Source: CAD feature listing. Evaluate the final solid. Frame: model axes, mm. A direction names the side the tool comes from. Give positions to 0.01 mm unless a question says otherwise; leave off trailing zeros. Order: outer loops, then holes, each group sorted by start corner. A loop starts at its lowest first (then second) coordinate and runs counter-clockwise, first axis right, second up. Notation, with made-up numbers: M 84.5,48.5 L 122.5,48.5 A10 cw 122.5,67.5 Z; hole C 26,32 d5. An arc over 180 degrees is marked long. Answer as a JSON object with one key per item and string values. Group by question number.
1. Pull-direction query (X, two-part tool) for faces 1 (the cylindrical face through (-9.918, 17.785, -252.536)), 2 (the flat face through (-8, 3, -85.725)), 3 (the cylindrical face through (-25.78, 18.78, -183.78)), 4 (the flat face through (4.445, 19, -248)); classes: +X half, -X half, draft (parallel to the pull), parting line (faces both ways), or undercut.
2. Material intervals for L1, parallel to X at y = 10, z = -203.2; L2, parallel to Z at x = -7, y = 4 (3 decimals); L3, parallel to X at y = 32, z = -1, sorted ascending. Write a range as [from, to].
3. Section query B-B (z = -203.2). Output: boundary loops of the cut face in (x, y), plus the area to 3 significant figures.
4. Section query D-D (y = 33). Output: boundary loops of the cut face in (x, z) (3 decimals), plus the area to 3 significant figures.
5. Section query C-C (x = 0). Output: boundary loops of the cut face in (y, z) (3 decimals), plus the area to 3 significant figures.
6. Section query A-A (y = 19.05). Output: boundary loops of the cut face in (x, z) (3 decimals), plus the area to 3 significant figures.
7. Set-up query: faces 5 (the flat face through (-4.445, 19, -248)), 6 (the flat face through (-15.24, 19, -260)), 7 (the flat face through (-4.762, 3, -67)). Return all of +Z, -Z, +X, -X, +Y, -Y with unobstructed straight access to the full face (end or side cutting, diameter ignored); none if empty.
8. Pin query (flat end, axial travel): P1, Ø5.5, axis at y = 2, z = -73, coming from the -X side; P2, Ø1, axis at y = 5.5, z = -170, coming from the +X side; P3, Ø8, axis at y = 18, z = -218.5, coming from the +X side. Return the tip coordinate at first contact, or that it passes through.
from build123d import *

# Parameters (mm, degrees)
SKETCH2_R           = 12.827
BOSS_EXTRUDE1_DEPTH = 38.1
CUT_EXTRUDE1_REACH  = 283.22
SKETCH3_R           = 3.302
SKETCH4_W           = 23.114
SKETCH4_H           = 31.75
CUT_EXTRUDE2_DEPTH  = 5.08
SKETCH5_W           = 9.525
SKETCH5_H           = 38.1
CUT_EXTRUDE3_DEPTH  = 5.08
CUT_EXTRUDE4_REACH  = 281.078
SKETCH6_W           = 6.604
SKETCH6_H           = 3.429


with BuildPart() as part:
    # Sketch2 → Boss-Extrude1 (new body)
    with BuildSketch(Plane(origin=(0, 0, 0), x_dir=(1, 0, 0), z_dir=(0, 1, 0))):
        with BuildLine():
            Line((-25.4, 0), (-25.4, 181.02040352))
            ThreePointArc((-25.4, 181.02040352), (-25.79242718, 183.816851484), (-26.939393939, 186.397275394))
            ThreePointArc((-26.939393939, 186.397275394), (-31.231288537, 208.915690363), (-19.242424242, 228.45453641))
            ThreePointArc((-19.242424242, 228.45453641), (-16.295425059, 232.026851209), (-15.24, 236.535988061))
            Line((-15.24, 236.535988061), (-15.24, 274.635988061))
            Line((-15.24, 274.635988061), (-4.445, 274.635988061))
            Line((-4.445, 274.635988061), (-4.445, 221.33211339))
            ThreePointArc((-4.445, 221.33211339), (0, 184.531), (4.445, 221.33211339))
            Line((4.445, 221.33211339), (4.445, 274.635988061))
            Line((4.445, 274.635988061), (15.24, 274.635988061))
            Line((15.24, 274.635988061), (15.24, 236.535988061))
            ThreePointArc((15.24, 236.535988061), (16.295425059, 232.026851209), (19.242424242, 228.45453641))
            ThreePointArc((19.242424242, 228.45453641), (31.231288537, 208.915690363), (26.939393939, 186.397275394))
            ThreePointArc((26.939393939, 186.397275394), (25.79242718, 183.816851484), (25.4, 181.02040352))
            Line((25.4, 181.02040352), (25.4, 0))
            ThreePointArc((25.4, 0), (0, -25.4), (-25.4, 0))
        make_face()
        with Locations(Location((0, 0, 0), (0, 0, 90))):
            Circle(SKETCH2_R, mode=Mode.SUBTRACT)
    extrude(amount=BOSS_EXTRUDE1_DEPTH)

    # Cut-Extrude1: up to this face of the body (flat: up to its plane)
    cut_extrude1_end = Plane(part.part.faces().sort_by_distance((15.24, 19.05, -255.585988061))[0])
    # Sketch3 → Cut-Extrude1 (cut, up to the picked face)
    with BuildSketch(Plane.ZY.offset(15.24), mode=Mode.PRIVATE) as cut_extrude1_sk1:
        with Locations((-255.585988061, 19.05)):
            Circle(SKETCH3_R)
    cut_extrude1_tool1 = split(extrude(cut_extrude1_sk1.sketch, amount=-CUT_EXTRUDE1_REACH, mode=Mode.PRIVATE), bisect_by=cut_extrude1_end, keep=Keep.BOTH, mode=Mode.PRIVATE)
    add(cut_extrude1_tool1.solids().sort_by(Axis((-15.24, 19.05, -255.585988), (1, 0, 0)))[0], mode=Mode.SUBTRACT)

    # Sketch4 → Cut-Extrude2 (cut)
    with BuildSketch(Plane.XZ):
        with Locations((0, -101.6)):
            Rectangle(SKETCH4_W, SKETCH4_H)
    extrude(amount=-CUT_EXTRUDE2_DEPTH, mode=Mode.SUBTRACT)

    # Sketch5 → Cut-Extrude3 (cut)
    with BuildSketch(Plane.XZ):
        with Locations((0, -66.675)):
            Rectangle(SKETCH5_W, SKETCH5_H)
    extrude(amount=-CUT_EXTRUDE3_DEPTH, mode=Mode.SUBTRACT)

    # Sketch6 → Cut-Extrude4 (cut, up to next)
    with BuildSketch(Plane.XZ, mode=Mode.PRIVATE) as cut_extrude4_sk1:
        with Locations((0, -14.109205523)):
            Rectangle(SKETCH6_W, SKETCH6_H)
    cut_extrude4_tool1 = extrude(cut_extrude4_sk1.sketch, amount=-CUT_EXTRUDE4_REACH, mode=Mode.PRIVATE) & part.part
    add(cut_extrude4_tool1.solids().sort_by_distance((0, 0, -14.109206))[0], mode=Mode.SUBTRACT)


solid = part.part
Answer sheet:
{
 "1": {"face 1": "draft", "face 2": "undercut", "face 3": "-X half", "face 4": "undercut"},
 "2": {"L1": "[-31.75, -18.67], [18.67, 31.75]", "L2": "[-274.636, -220.507], [-185.893, -117.475], [-85.725, -10.749], [10.749, 24.416]", "L3": "[-25.4, -12.79], [12.79, 25.4]"},
 "3": {"outline": "M -31.75,0 L -18.67,0 L -18.67,38.1 L -31.75,38.1 Z; M 18.67,0 L 31.75,0 L 31.75,38.1 L 18.67,38.1 Z", "area": "997 mm^2"},
 "4": {"outline": "M -26.939,-186.397 A31.75 ccw -19.242,-228.455 A10.16 cw -15.24,-236.536 L -15.24,-274.636 L -4.445,-274.636 L -4.445,-221.332 A18.669 cw long 4.445,-221.332 L 4.445,-274.636 L 15.24,-274.636 L 15.24,-236.536 A10.16 cw 19.242,-228.455 A31.75 ccw 26.939,-186.397 A10.16 cw 25.4,-181.02 L 25.4,0 A25.4 ccw -25.4,0 L -25.4,-181.02 A10.16 cw Z; hole M -3.302,-15.824 L 3.302,-15.824 L 3.302,-12.395 A12.827 ccw long -3.302,-12.395 Z", "area": "12,200 mm^2"},
 "5": {"outline": "M 0,-184.531 L 38.1,-184.531 L 38.1,-15.824 L 0,-15.824 L 0,-47.625 L 5.08,-47.625 L 5.08,-117.475 L 0,-117.475 Z; M 0,12.827 L 38.1,12.827 L 38.1,25.4 L 0,25.4 Z", "area": "6,550 mm^2"},
 "6": {"outline": "M -26.939,-186.397 A31.75 ccw -19.242,-228.455 A10.16 cw -15.24,-236.536 L -15.24,-252.284 L -4.445,-252.284 L -4.445,-221.332 A18.669 cw long 4.445,-221.332 L 4.445,-252.284 L 15.24,-252.284 L 15.24,-236.536 A10.16 cw 19.242,-228.455 A31.75 ccw 26.939,-186.397 A10.16 cw 25.4,-181.02 L 25.4,0 A25.4 ccw -25.4,0 L -25.4,-181.02 A10.16 cw Z; M -15.24,-274.636 L -4.445,-274.636 L -4.445,-258.888 L -15.24,-258.888 Z; M 4.445,-274.636 L 15.24,-274.636 L 15.24,-258.888 L 4.445,-258.888 Z; hole M -3.302,-15.824 L 3.302,-15.824 L 3.302,-12.395 A12.827 ccw long -3.302,-12.395 Z", "area": "12,100 mm^2"},
 "7": {"face 5": "-Z, +Y, -Y", "face 6": "-Z, -X, +Y, -Y", "face 7": "-Y"},
 "8": {"P1": "x = -25.4", "P2": "x = 25.4", "P3": "x = 29.67"}
}
